Could you check a few things on this drawing? It's one solid part, dimensions in mm from its lowest x, y, z. Give positions to 0.01 mm unless a question says otherwise; leave off trailing zeros. Order: outer loops, then holes, each group sorted by start corner. A loop starts at its lowest first (then second) coordinate and runs counter-clockwise, first axis right, second up.
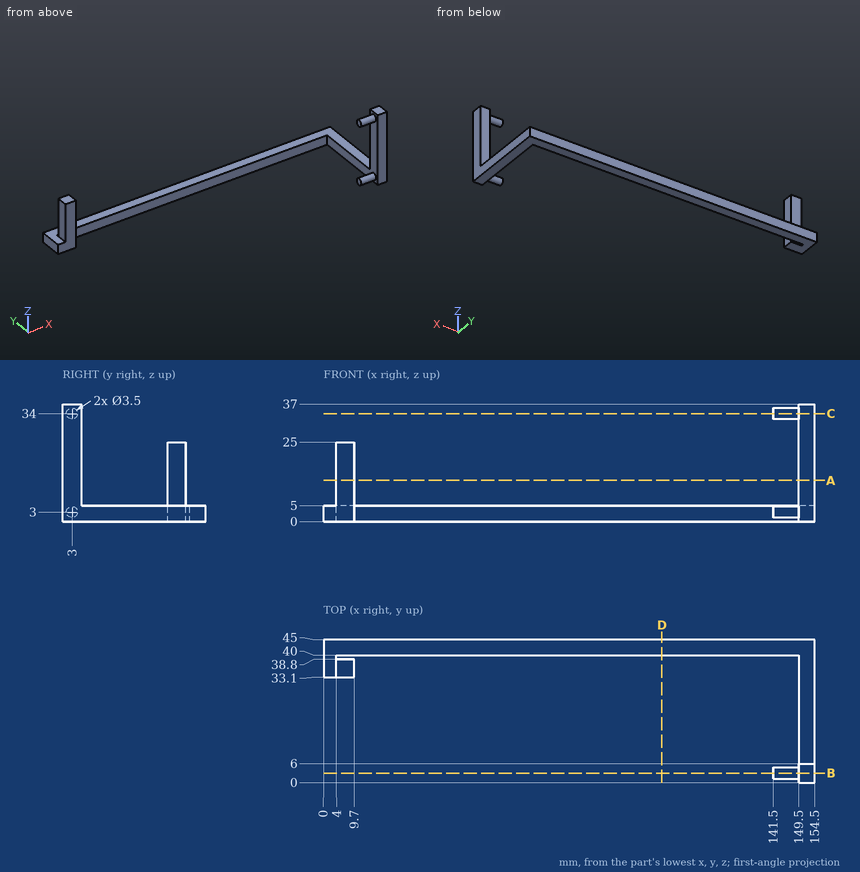
Item 1: Imagine slicing it at C-C on z = 34. List the corners of the cut face in (x, y) for me, then the cut area to 3 significant figures.
Findings:
outline: (141.5, 1.25) - (149.5, 1.25) - (149.5, 0) - (154.5, 0) - (154.5, 6) - (149.5, 6) - (149.5, 4.75) - (141.5, 4.75) - close
area: 58.0 mm2
Item 2: Please list where these lines run through material, in increasing order: line 1 along Z through (x, y) = (30, 41); line 2 along X through (y, z) = (3.5, 34.5); line 3 along X through (y, z) = (5, 6.5).
Findings:
line 1: z = 0 to 5
line 2: x = 141.5 to 154.5
line 3: x = 149.5 to 154.5
Item 3: Imagine slicing it at B-B on y = 3. List the corners of the cut face in (x, z) for me.
Findings:
outline: (141.5, 1.25) - (149.5, 1.25) - (149.5, 0) - (154.5, 0) - (154.5, 37) - (149.5, 37) - (149.5, 35.75) - (141.5, 35.75) - (141.5, 32.25) - (149.5, 32.25) - (149.5, 4.75) - (141.5, 4.75) - close
Item 4: For pin 1 (11 mm diameter, centred on y = 23, z = 18, fed in from -X); pin 2 (1.7 mm diameter, centred on y = 34.5, z = 10.5, fed in from -X); pin 3 (8 mm diameter, centred on y = 33.5, z = 19, fed in from +X); pin 4 (1.5 mm diameter, centred on x = 104, z = 3.5, fed in from -Y), each with a flat end and sliding along its axis, tell me the tip position at first contact or that it passes through.
Findings:
pin 1: passes through
pin 2: stops at x = 4
pin 3: stops at x = 9.7
pin 4: stops at y = 40
Item 5: Imagine slicing it at D-D on x = 106.5. List the corners of the cut face in (y, z) for me, then the cut area to 3 significant figures.
Findings:
outline: (40, 0) - (45, 0) - (45, 5) - (40, 5) - close
area: 25.0 mm2
Item 6: Imagine slicing it at A-A on z = 13. List the corners of the cut face in (x, y) for me.
Findings:
outline: (4, 33.1) - (9.7, 33.1) - (9.7, 38.8) - (4, 38.8) - close; (149.5, 0) - (154.5, 0) - (154.5, 6) - (149.5, 6) - close
